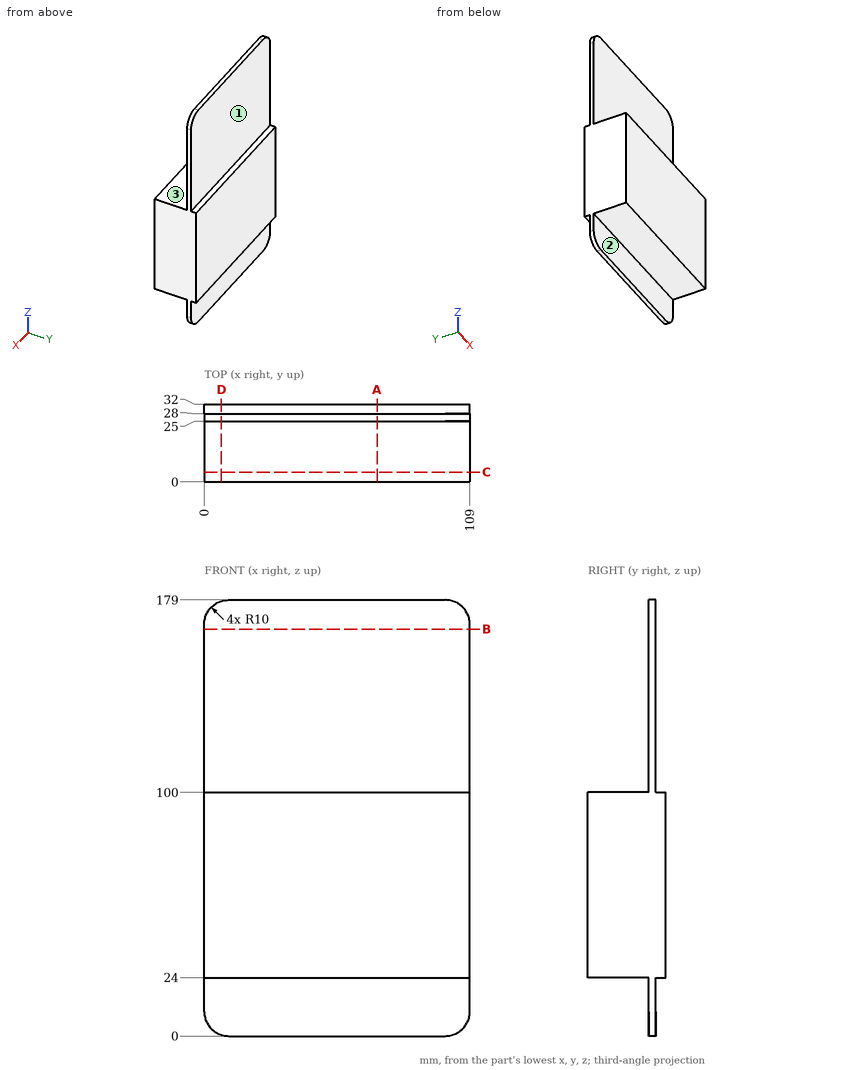
Design review of the part shown in the three views and the two pictorial views. Dimensions are in mm from the part's minimum x, y and z. A direction names the side the tool comes from. Round coordinates to 2 decimals unless told otherwise and drop trailing zeros. Loops run counter-clockwise (first coordinate to the right, second up) from the corner with the lowest first, then second, coordinate; pieces in that order, holes last. Notation, with made-up numbers: (89, 38.25) -> (120, 38.25) arc R26 cw to (120, 61.25) -> close; hole circle Ø6 at (53.5, -16.75). An arc over 180 degrees is marked (long way). Return JSON: item names as keys, results as strings.
(1) Add section A-A on x = 71. Write out the cut boundary in (y, z), plus the area to 3 significant figures.
Solved:
{"outline": "(0, 24) -> (25, 24) -> (25, 0) -> (28, 0) -> (28, 24) -> (32, 24) -> (32, 100) -> (28, 100) -> (28, 179) -> (25, 179) -> (25, 100) -> (0, 100) -> close", "area": "2,740 mm2"}
(2) For pin 1 (4 mm diameter, centred on x = 76.5, y = 19, fed in from +Z); pin 2 (6 mm diameter, centred on x = 91, y = 20.5, fed in from -Z); pin 3 (23.5 mm diameter, centred on x = 43.5, z = 143.5, fed in from +Y); pin 4 (2 mm diameter, centred on x = 68.5, z = 72.5, fed in from -Y), all flat-tipped, find the tip position at first contact; note any pin that passes through.
Solved:
{"pin 1": "z = 100", "pin 2": "z = 24", "pin 3": "y = 28", "pin 4": "y = 0"}
(3) Add section D-D on x = 7. Write out the cut boundary in (y, z), plus the area to 3 significant figures.
Solved:
{"outline": "(0, 24) -> (25, 24) -> (25, 0.46) -> (28, 0.46) -> (28, 24) -> (32, 24) -> (32, 100) -> (28, 100) -> (28, 178.54) -> (25, 178.54) -> (25, 100) -> (0, 100) -> close", "area": "2,740 mm2"}
(4) Add section C-C on y = 4. Write out the cut boundary in (x, z), plus the area to 3 significant figures.
Solved:
{"outline": "(0, 24) -> (109, 24) -> (109, 100) -> (0, 100) -> close", "area": "8,280 mm2"}
(5) Add section B-B on z = 167. Write out the cut boundary in (x, y), plus the area to 3 significant figures.
Solved:
{"outline": "(0, 25) -> (109, 25) -> (109, 28) -> (0, 28) -> close", "area": "327 mm2"}
(6) For line 1 (Y direction, x = 30, z = 157); line 2 (Z direction, x = 74, y = 6.5), list the stretches that pass through material, from the lowest coordinate up.
Solved:
{"line 1": "25 to 28", "line 2": "24 to 100"}
(7) For the marked faces 1, 2 and 3, list the 3-axis set-ups (+Z, -Z, +X, -X, +Y, -Y) from which the entire face can be reached by the end or side of a thin tool; tool diameter is ignored.
Solved:
{"face 1": "+Z, +X, -X, +Y", "face 2": "-Z, +X, -X, -Y", "face 3": "+Z, +X, -X, -Y"}
